from build123d import *

# Parameters (mm, degrees)
F0_W     = 25.4
F0_H     = 25.4
F0_W_2   = 22.225
F0_H_2   = 22.225
F1_DEPTH = 101.6
F2_R     = 1.5875
F3_DEPTH = 25.4
F5_DEPTH = 25.4


with BuildPart() as f1:
    # F0 (on Top) → F1 (new body)
    with BuildSketch(Plane.XY):
        Rectangle(F0_W, F0_H)
        Rectangle(F0_W_2, F0_H_2, mode=Mode.SUBTRACT)
    extrude(amount=F1_DEPTH)

    # F2 (on face) → F3 (cut)
    with BuildSketch(Plane.XZ.offset(12.7)):
        with BuildLine():
            ThreePointArc((1.5875, 95.25), (1.122532, 96.372532), (0, 96.8375))
            Line((0, 96.8375), (0, 93.6625))
            ThreePointArc((0, 93.6625), (1.122532, 94.127468), (1.5875, 95.25))
        make_face()
        with BuildLine():
            ThreePointArc((1.5875, 6.35), (1.122532, 7.472532), (0, 7.9375))
            Line((0, 7.9375), (0, 4.7625))
            ThreePointArc((0, 4.7625), (1.122532, 5.227468), (1.5875, 6.35))
        make_face()
        with BuildLine():
            Line((0, 4.7625), (0, 7.9375))
            ThreePointArc((0, 7.9375), (-1.5875, 6.35), (0, 4.7625))
        make_face()
        with BuildLine():
            ThreePointArc((1.5875, 19.05), (1.122532, 20.172532), (0, 20.6375))
            Line((0, 20.6375), (0, 17.4625))
            ThreePointArc((0, 17.4625), (1.122532, 17.927468), (1.5875, 19.05))
        make_face()
        with BuildLine():
            Line((0, 17.4625), (0, 20.6375))
            ThreePointArc((0, 20.6375), (-1.5875, 19.05), (0, 17.4625))
        make_face()
        with BuildLine():
            ThreePointArc((1.5875, 31.75), (1.122532, 32.872532), (0, 33.3375))
            Line((0, 33.3375), (0, 30.1625))
            ThreePointArc((0, 30.1625), (1.122532, 30.627468), (1.5875, 31.75))
        make_face()
        with BuildLine():
            Line((0, 30.1625), (0, 33.3375))
            ThreePointArc((0, 33.3375), (-1.5875, 31.75), (0, 30.1625))
        make_face()
        with BuildLine():
            ThreePointArc((1.5875, 44.45), (1.122532, 45.572532), (0, 46.0375))
            Line((0, 46.0375), (0, 42.8625))
            ThreePointArc((0, 42.8625), (1.122532, 43.327468), (1.5875, 44.45))
        make_face()
        with BuildLine():
            Line((0, 42.8625), (0, 46.0375))
            ThreePointArc((0, 46.0375), (-1.5875, 44.45), (0, 42.8625))
        make_face()
        with BuildLine():
            ThreePointArc((1.5875, 57.15), (1.122532, 58.272532), (0, 58.7375))
            Line((0, 58.7375), (0, 55.5625))
            ThreePointArc((0, 55.5625), (1.122532, 56.027468), (1.5875, 57.15))
        make_face()
        with BuildLine():
            Line((0, 55.5625), (0, 58.7375))
            ThreePointArc((0, 58.7375), (-1.5875, 57.15), (0, 55.5625))
        make_face()
        with BuildLine():
            ThreePointArc((1.5875, 69.85), (1.122532, 70.972532), (0, 71.4375))
            Line((0, 71.4375), (0, 68.2625))
            ThreePointArc((0, 68.2625), (1.122532, 68.727468), (1.5875, 69.85))
        make_face()
        with BuildLine():
            Line((0, 68.2625), (0, 71.4375))
            ThreePointArc((0, 71.4375), (-1.5875, 69.85), (0, 68.2625))
        make_face()
        with BuildLine():
            ThreePointArc((1.5875, 82.55), (1.122532, 83.672532), (0, 84.1375))
            Line((0, 84.1375), (0, 80.9625))
            ThreePointArc((0, 80.9625), (1.122532, 81.427468), (1.5875, 82.55))
        make_face()
        with BuildLine():
            Line((0, 80.9625), (0, 84.1375))
            ThreePointArc((0, 84.1375), (-1.5875, 82.55), (0, 80.9625))
        make_face()
        with BuildLine():
            Line((0, 93.6625), (0, 96.8375))
            ThreePointArc((0, 96.8375), (-1.5875, 95.25), (0, 93.6625))
        make_face()
        with Locations((92.636349, -11.009342)):
            Circle(F2_R)
        with Locations((123.515132, -46.429122)):
            Circle(F2_R)
    extrude(amount=-F3_DEPTH, mode=Mode.SUBTRACT)

    # F4 (on face) → F5 (cut)
    with BuildSketch(Plane.YZ.offset(12.7)):
        with BuildLine():
            ThreePointArc((1.5875, 95.25), (1.122532, 96.372532), (0, 96.8375))
            Line((0, 96.8375), (0, 93.6625))
            ThreePointArc((0, 93.6625), (1.122532, 94.127468), (1.5875, 95.25))
        make_face()
        with BuildLine():
            ThreePointArc((1.5875, 6.35), (1.122532, 7.472532), (0, 7.9375))
            Line((0, 7.9375), (0, 4.7625))
            ThreePointArc((0, 4.7625), (1.122532, 5.227468), (1.5875, 6.35))
        make_face()
        with BuildLine():
            Line((0, 4.7625), (0, 7.9375))
            ThreePointArc((0, 7.9375), (-1.5875, 6.35), (0, 4.7625))
        make_face()
        with BuildLine():
            ThreePointArc((1.5875, 19.05), (1.122532, 20.172532), (0, 20.6375))
            Line((0, 20.6375), (0, 17.4625))
            ThreePointArc((0, 17.4625), (1.122532, 17.927468), (1.5875, 19.05))
        make_face()
        with BuildLine():
            Line((0, 17.4625), (0, 20.6375))
            ThreePointArc((0, 20.6375), (-1.5875, 19.05), (0, 17.4625))
        make_face()
        with BuildLine():
            ThreePointArc((1.5875, 31.75), (1.122532, 32.872532), (0, 33.3375))
            Line((0, 33.3375), (0, 30.1625))
            ThreePointArc((0, 30.1625), (1.122532, 30.627468), (1.5875, 31.75))
        make_face()
        with BuildLine():
            Line((0, 30.1625), (0, 33.3375))
            ThreePointArc((0, 33.3375), (-1.5875, 31.75), (0, 30.1625))
        make_face()
        with BuildLine():
            ThreePointArc((1.5875, 44.45), (1.122532, 45.572532), (0, 46.0375))
            Line((0, 46.0375), (0, 42.8625))
            ThreePointArc((0, 42.8625), (1.122532, 43.327468), (1.5875, 44.45))
        make_face()
        with BuildLine():
            Line((0, 42.8625), (0, 46.0375))
            ThreePointArc((0, 46.0375), (-1.5875, 44.45), (0, 42.8625))
        make_face()
        with BuildLine():
            ThreePointArc((1.5875, 57.15), (1.122532, 58.272532), (0, 58.7375))
            Line((0, 58.7375), (0, 55.5625))
            ThreePointArc((0, 55.5625), (1.122532, 56.027468), (1.5875, 57.15))
        make_face()
        with BuildLine():
            Line((0, 55.5625), (0, 58.7375))
            ThreePointArc((0, 58.7375), (-1.5875, 57.15), (0, 55.5625))
        make_face()
        with BuildLine():
            ThreePointArc((1.5875, 69.85), (1.122532, 70.972532), (0, 71.4375))
            Line((0, 71.4375), (0, 68.2625))
            ThreePointArc((0, 68.2625), (1.122532, 68.727468), (1.5875, 69.85))
        make_face()
        with BuildLine():
            Line((0, 68.2625), (0, 71.4375))
            ThreePointArc((0, 71.4375), (-1.5875, 69.85), (0, 68.2625))
        make_face()
        with BuildLine():
            ThreePointArc((1.5875, 82.55), (1.122532, 83.672532), (0, 84.1375))
            Line((0, 84.1375), (0, 80.9625))
            ThreePointArc((0, 80.9625), (1.122532, 81.427468), (1.5875, 82.55))
        make_face()
        with BuildLine():
            Line((0, 80.9625), (0, 84.1375))
            ThreePointArc((0, 84.1375), (-1.5875, 82.55), (0, 80.9625))
        make_face()
        with BuildLine():
            Line((0, 93.6625), (0, 96.8375))
            ThreePointArc((0, 96.8375), (-1.5875, 95.25), (0, 93.6625))
        make_face()
    extrude(amount=-F5_DEPTH, mode=Mode.SUBTRACT)


solid = f1.part
Can you work these out from the model? Positions are in its coordinate system, mm. A direction names the side the tool comes from. Give positions to 0.01 mm unless a question says otherwise; leave off trailing zeros. Write each loop counter-clockwise with the first axis right and the second up, starting at its lowest first coordinate (ties: lowest second). Pieces come first, ordered by that corner, then holes. Notation, with made-up numbers: M 5.5,-29.5 L 48.5,-29.5 A30 cw 48.5,7.5 Z; hole C -36,-34 d11. An arc over 180 degrees is marked long. Answer in a Markdown table with one row per item. Add a question column.
Item 1: Imagine slicing it at A-A, the plane y = -6.75. Write out the boundary of the cut face in (x, z).
Item 2: We'd pull the mould along X, two halves only. Please class faces 1 (the flat face through (0, 11.112, 50)), 2 (the flat face through (0, -12.7, 50)), 3 (the flat face through (12.7, 0, 50)): released by +X, released by -X, zero draft, split by the parting line, or undercut.
Item 3: On a 3-axis mill with a long thin cutter (end or side, diameter ignored), from which of +Z, -Z, +X, -X, +Y, -Y can I reach the whole of each face in a straight line? I mean faces 4 (the flat face through (0, 12.7, 50)), 5 (the flat face through (0, -11.112, 50)). Say none if no direction works.
Item 4: Please list where these lines run through material, in increasing order: L1, parallel to Y at x = -0.25, z = 52.5; L2, parallel to X at y = 11.5, z = 18.5.
Item 5: Imagine slicing it at C-C, the plane z = 92. Write out the boundary of the cut face in (x, y), plus the area to 3 significant figures.
Evaluation:
| question | item | result |
|---|---|---|
| 1 | outline | M -12.7,0 L -11.11,0 L -11.11,101.6 L -12.7,101.6 Z; M 11.11,0 L 12.7,0 L 12.7,101.6 L 11.11,101.6 Z |
| 2 | face 1 | undercut |
| 2 | face 2 | zero draft |
| 2 | face 3 | released by +X |
| 3 | face 4 | +Z, -Z, +X, -X, +Y |
| 3 | face 5 | +Z, -Z |
| 4 | L1 | y = -12.7 to -11.11, 11.11 to 12.7 |
| 4 | L2 | x = -12.7 to -1.49, 1.49 to 12.7 |
| 5 | outline | M -12.7,-12.7 L 12.7,-12.7 L 12.7,12.7 L -12.7,12.7 Z; hole M -11.11,-11.11 L 11.11,-11.11 L 11.11,11.11 L -11.11,11.11 Z |
| 5 | area | 151 mm² |
